Could you check a few things on this drawing? It's one solid part, dimensions in mm from its lowest x, y, z. A direction names the side the tool comes from. Give positions to 0.01 mm unless a question says otherwise; leave off trailing zeros. Order: outer loops, then holes, each group sorted by start corner. A loop starts at its lowest first (then second) coordinate and runs counter-clockwise, first axis right, second up. Notation, with made-up numbers: (79, -32) -> (117, -32) arc R29 ccw to (117, 2) -> close; hole circle Ø3 at (57, -35). An arc over 180 degrees is marked (long way). Write each question's results on one line, items separated by ' | '.
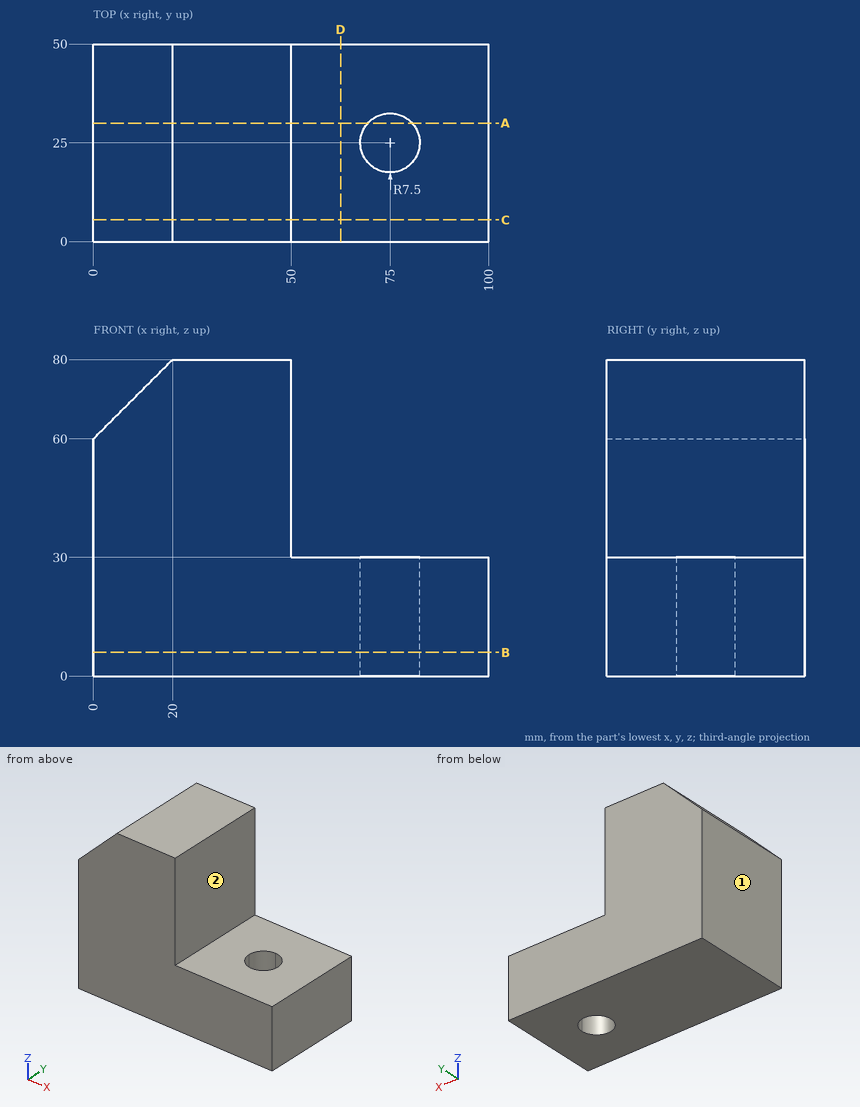
Q1. For the marked faces 1 and 2, which set-ups out of +Z, -Z, +X, -X, +Y, -Y let a thin tool reach every point of the face, with its end or its side?
Here are the results:
face 1: +Z, -Z, -X, +Y, -Y | face 2: +Z, +X, +Y, -Y
Q2. Suppose I cut it at C-C on y = 5.5. Please give me the cut outline in (x, z), and give its area (3 significant figures).
Here are the results:
outline: (0, 0) -> (100, 0) -> (100, 30) -> (50, 30) -> (50, 80) -> (20, 80) -> (0, 60) -> close | area: 5,300 mm²
Q3. I'm going to push flat-ended pins straight in: pin 1 Ø1 at (x, y) = (51, 11) entering from +Z; pin 2 Ø1 at (y, z) = (7, 57.5) entering from +X; pin 3 Ø2 at (x, y) = (38.5, 19) entering from -Z; pin 4 Ø6 at (y, z) = (30, 68.5) entering from -X. Where does each tip first touch, or does it pass through?
Here are the results:
pin 1: stops at z = 30 | pin 2: stops at x = 50 | pin 3: stops at z = 0 | pin 4: stops at x = 5.5
Q4. Suppose I cut it at D-D on x = 62.5. Please give me the cut outline in (y, z).
Here are the results:
outline: (0, 0) -> (50, 0) -> (50, 30) -> (0, 30) -> close
Q5. Suppose I cut it at B-B on z = 6. Please give me the cut outline in (x, y), and give its area (3 significant figures).
Here are the results:
outline: (0, 0) -> (100, 0) -> (100, 50) -> (0, 50) -> close; hole circle Ø15 at (75, 25) | area: 4,820 mm²
Q6. Suppose I cut it at A-A on y = 30. Please give me the cut outline in (x, z).
Here are the results:
outline: (0, 0) -> (69.41, 0) -> (69.41, 30) -> (50, 30) -> (50, 80) -> (20, 80) -> (0, 60) -> close; (80.59, 0) -> (100, 0) -> (100, 30) -> (80.59, 30) -> close
Q7. I need wall thicknesses on line 1 along X through (y, z) = (19, 33); line 2 along Z through (x, y) = (56, 7); line 3 along X through (y, z) = (23, 26.5). Which ranges of each line are inside material? Lowest first, please.
Here are the results:
line 1: x = 0 to 50 | line 2: z = 0 to 30 | line 3: x = 0 to 67.77, 82.23 to 100
